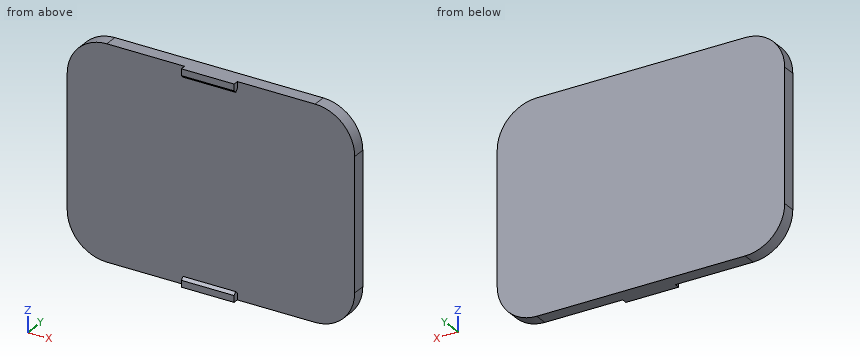
from build123d import *

# Parameters (mm, degrees)
BOSS_EXTRUDE1_DEPTH = 5
BOSS_EXTRUDE2_DEPTH = 10


with BuildPart() as part:
    # Sketch1 → Boss-Extrude1 (new body)
    with BuildSketch(Plane(origin=(0, 0, 0), x_dir=(1, 0, 0), z_dir=(0, 1, 0))):
        with BuildLine():
            Line((-39.5, 40), (39.5, 40))
            ThreePointArc((39.5, 40), (50.106601718, 35.606601718), (54.5, 25))
            Line((54.5, 25), (54.5, -25))
            ThreePointArc((54.5, -25), (50.106601718, -35.606601718), (39.5, -40))
            Line((39.5, -40), (-39.5, -40))
            ThreePointArc((-39.5, -40), (-50.106601718, -35.606601718), (-54.5, -25))
            Line((-54.5, -25), (-54.5, 25))
            ThreePointArc((-54.5, 25), (-50.106601718, 35.606601718), (-39.5, 40))
        make_face()
    extrude(amount=BOSS_EXTRUDE1_DEPTH)

    # Sketch2 → Boss-Extrude2 (add, symmetric)
    with BuildSketch(Plane(origin=(0, 0, 0), x_dir=(0, 0, -1), z_dir=(1, 0, 0))):
        Polygon((-37.5, 0), (-40, 0), (-40, -2), (-37.5, -2), (-36.5, -1), align=None)
    boss_extrude2 = extrude(amount=BOSS_EXTRUDE2_DEPTH, both=True)

    # Mirror1: Boss-Extrude2 across plane
    add(boss_extrude2.mirror(Plane.XY))


solid = part.part
Here's how the part is built. I have some questions about the finished solid (model axes, mm). Round coordinates to 2 decimals unless told otherwise and drop trailing zeros. Write each loop counter-clockwise with the first axis right and the second up, starting at its lowest first coordinate (ties: lowest second). Pieces come first, ordered by that corner, then holes. Notation, with made-up numbers: (86, 20) -> (100, 20) arc R29 ccw to (100, 50) -> close; hole circle Ø3 at (83, 25.5). An arc over 180 degrees is marked (long way). One line per item, written item: value.
1) Suppose I cut it at D-D on x = -16.5. List the corners of the cut face in (y, z) for me.
Filled sheet:
outline: (0, -40) -> (5, -40) -> (5, 40) -> (0, 40) -> close
2) If I drill on line 1 (Y direction, x = 14, z = -6); line 2 (Z direction, x = -0.5, y = -0.5); line 3 (Z direction, x = 47.5, y = 4), over which ranges is the centre line in solid material (lowest first)? Write a range as [from, to].
Filled sheet:
line 1: y = [0, 5]
line 2: z = [-40, -37], [37, 40]
line 3: z = [-37.69, 37.69]
3) Suppose I cut it at A-A on x = -2.5. List the corners of the cut face in (y, z) for me.
Filled sheet:
outline: (-2, -40) -> (5, -40) -> (5, 40) -> (-2, 40) -> (-2, 37.5) -> (-1, 36.5) -> (0, 37.5) -> (0, -37.5) -> (-1, -36.5) -> (-2, -37.5) -> close
4) Suppose I cut it at B-B on y = 2.25. List the corners of the cut face in (x, z) for me, plus the area to 3 significant figures.
Filled sheet:
outline: (-54.5, -25) arc R15 ccw to (-39.5, -40) -> (39.5, -40) arc R15 ccw to (54.5, -25) -> (54.5, 25) arc R15 ccw to (39.5, 40) -> (-39.5, 40) arc R15 ccw to (-54.5, 25) -> close
area: 8,530 mm2
5) Suppose I cut it at C-C on z = 5. List the corners of the cut face in (x, y) for me.
Filled sheet:
outline: (-54.5, 0) -> (54.5, 0) -> (54.5, 5) -> (-54.5, 5) -> close
6) I'm going to push flat-ended pins straight in: pin 1 Ø0.6 at (y, z) = (-1.5, -38) entering from +X; pin 2 Ø24 at (x, z) = (-5.5, 5.5) entering from -Y; pin 3 Ø1 at (y, z) = (-1, -38) entering from -X. Where does each tip first touch, or does it pass through?
Filled sheet:
pin 1: stops at x = 10
pin 2: stops at y = 0
pin 3: stops at x = -10
